For this review, take the finished solid that the model builds, in its own axes (mm). Face numbers are marked on the shaded views. A direction names the side the tool comes from. Coordinates: 2 decimals unless noted, no trailing zeros. Order: outer loops, then holes, each group sorted by start corner. A loop starts at its lowest first (then second) coordinate and runs counter-clockwise, first axis right, second up. Notation, with made-up numbers: M -6,-34.5 L 26,-34.5 A29 ccw 26,-13.5 Z; hole C 10.25,8.5 d3. An arc over 180 degrees is marked long. Use one line per item in the form item = value. Start each with the question number.
```python
from build123d import *

# Parameters (mm, degrees)
SZKIC1_W                    = 7
SZKIC1_H                    = 6
DODANIE_WYCI_GNI_CIE1_DEPTH = 0.25
SZKIC2_W                    = 7
SZKIC2_H                    = 4
DODANIE_WYCI_GNI_CIE2_DEPTH = 1.25
SZKIC3_W                    = 7
SZKIC3_H                    = 6
DODANIE_WYCI_GNI_CIE3_DEPTH = 0.5
SZKIC4_R                    = 2
DODANIE_WYCI_GNI_CIE4_DEPTH = 1.5
ZAOKR_GLENIE1_R             = 0.25
ZAOKR_GLENIE2_R             = 1
SZKIC5_W                    = 4
SZKIC5_H                    = 1
DODANIE_WYCI_GNI_CIE5_DEPTH = 1
SZKIC6_W                    = 2
SZKIC6_H                    = 0.25
WYTNIJ_WYCI_GNI_CIE1_DEPTH  = 1


with BuildPart() as part:
    # Szkic1 → Dodanie-wyciągnięcie1 (new body)
    with BuildSketch(Plane(origin=(0, 0, 0), x_dir=(1, 0, 0), z_dir=(0, 1, 0))):
        Rectangle(SZKIC1_W, SZKIC1_H)
    extrude(amount=DODANIE_WYCI_GNI_CIE1_DEPTH)

    # Szkic2 → Dodanie-wyciągnięcie2 (add)
    with BuildSketch(Plane(origin=(0, 0.25, 0), x_dir=(1, 0, 0), z_dir=(0, 1, 0))):
        Rectangle(SZKIC2_W, SZKIC2_H)
    extrude(amount=DODANIE_WYCI_GNI_CIE2_DEPTH)

    # Szkic3 → Dodanie-wyciągnięcie3 (add)
    with BuildSketch(Plane(origin=(0, 1.5, 0), x_dir=(1, 0, 0), z_dir=(0, 1, 0))):
        Rectangle(SZKIC3_W, SZKIC3_H)
    extrude(amount=DODANIE_WYCI_GNI_CIE3_DEPTH)

    # Szkic4 → Dodanie-wyciągnięcie4 (add)
    with BuildSketch(Plane(origin=(0, 2, 0), x_dir=(1, 0, 0), z_dir=(0, 1, 0))):
        with Locations(Location((0, 0, 0), (0, 0, 270))):
            Circle(SZKIC4_R)
    extrude(amount=DODANIE_WYCI_GNI_CIE4_DEPTH)

    # Zaokrąglenie1
    zaokr_glenie1_edges = [part.edges().sort_by_distance(p)[0] for p in [
        (0, 2, -2),
        (0, 3.5, -2),
    ]]
    fillet(zaokr_glenie1_edges, radius=ZAOKR_GLENIE1_R)

    # Zaokrąglenie2
    zaokr_glenie2_edges = [part.edges().sort_by_distance(p)[0] for p in [
        (-3.5, 1.75, -3),
        (3.5, 1.75, -3),
        (3.5, 1.75, 3),
        (-3.5, 1.75, 3),
    ]]
    fillet(zaokr_glenie2_edges, radius=ZAOKR_GLENIE2_R)

    # Szkic5 → Dodanie-wyciągnięcie5 (add)
    with BuildSketch(Plane.XZ):
        Rectangle(SZKIC5_W, SZKIC5_H)
    extrude(amount=DODANIE_WYCI_GNI_CIE5_DEPTH)

    # Szkic6 → Wytnij-wyciągnięcie1 (cut)
    with BuildSketch(Plane(origin=(0, 0, -0.5), x_dir=(-1, 0, 0), z_dir=(0, 0, -1))):
        with Locations((0, -0.375)):
            Rectangle(SZKIC6_W, SZKIC6_H)
    extrude(amount=-WYTNIJ_WYCI_GNI_CIE1_DEPTH, mode=Mode.SUBTRACT)


solid = part.part
```
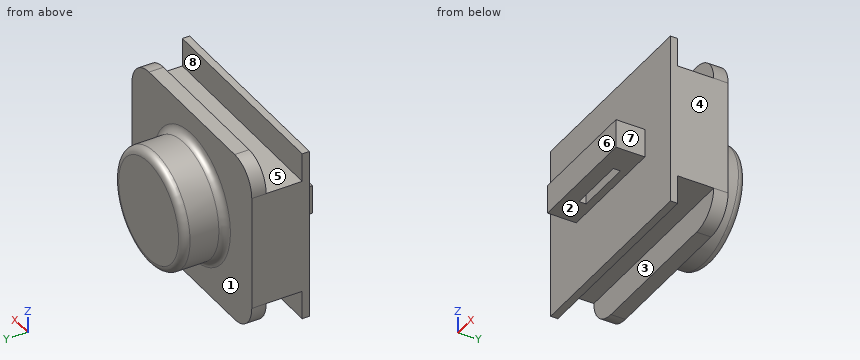
1. To check wall thickness, follow line 1 (Y direction, x = 1, z = -2.25); line 2 (Y direction, x = 0, z = -0.25); line 3 (Y direction, x = -0.25, z = 1.55). State the ranges of each line that lie inside material, in increasing order.
2. Consider section B-B, the plane y = 1.75. Write out the cut boundary in (x, z), plus the area to 3 significant figures.
3. The part is to be moulded in two halves that separate along Y. For the marked faces 6, 7 and 8, say which applies: pulls with the +Y half, pulls with the -Y half, needs draft (parallel to the pull), parting line crosses it, or undercut.
4. Consider section C-C, the plane z = 0. Write out the cut boundary in (x, y), plus the area to 3 significant figures.
5. Tool access review of the marked faces 1, 2, 3, 4 and 5: name each direction out of +Z, -Z, +X, -X, +Y, -Y from which nothing blocks a thin tool from reaching the whole face with its end or side.
6. Consider section A-A, the plane x = 0. Write out the cut boundary in (y, z).
7. For pin 1 Ø0.8 at (x, z) = (0, 2.5) entering from -Y; pin 2 Ø1 at (x, y) = (-1.5, 0.5) entering from +Z; pin 3 Ø0.8 at (x, y) = (1, -0.5) entering from -Z; pin 4 Ø0.8 at (x, z) = (1.5, 2.5) entering from +Y, all flat-tipped, find the tip position at first contact; note any pin that passes through.
8. Consider section D-D, the plane z = 2.4. Write out the cut boundary in (x, y), plus the area to 3 significant figures.
Answers follow:
q1.line_1 = 0 to 0.25, 1.5 to 2
q1.line_2 = -1 to -0.5, -0.25 to 3.5
q1.line_3 = 0 to 3.5
q2.outline = M -3.5,-2 A1 ccw -2.5,-3 L 2.5,-3 A1 ccw 3.5,-2 L 3.5,2 A1 ccw 2.5,3 L -2.5,3 A1 ccw -3.5,2 Z
q2.area = 41.1 mm²
q3.face_6 = pulls with the -Y half
q3.face_7 = needs draft
q3.face_8 = undercut
q4.outline = M -3.5,0 L -2,0 L -2,-1 L 2,-1 L 2,0 L 3.5,0 L 3.5,2 L 2.25,2 A0.25 cw 2,2.25 L 2,3.25 A0.25 ccw 1.75,3.5 L -1.75,3.5 A0.25 ccw -2,3.25 L -2,2.25 A0.25 cw -2.25,2 L -3.5,2 Z; hole M -1,-0.5 L 1,-0.5 L 1,-0.25 L -1,-0.25 Z
q4.area = 23.5 mm²
q5.face_1 = +Y
q5.face_2 = -Z, +X, -X, -Y
q5.face_3 = -Z, +X, -X
q5.face_4 = +Z, -Z, +X, +Y, -Y
q5.face_5 = +Z, +X, -X
q6.outline = M -1,-0.5 L -0.5,-0.5 L -0.5,0.5 L -1,0.5 Z; M -0.25,-0.5 L 0,-0.5 L 0,-3 L 0.25,-3 L 0.25,-2 L 1.5,-2 L 1.5,-3 L 2,-3 L 2,-2.25 A0.25 cw 2.25,-2 L 3.25,-2 A0.25 ccw 3.5,-1.75 L 3.5,1.75 A0.25 ccw 3.25,2 L 2.25,2 A0.25 cw 2,2.25 L 2,3 L 1.5,3 L 1.5,2 L 0.25,2 L 0.25,3 L 0,3 L 0,0.5 L -0.25,0.5 Z
q7.pin_1 = 0
q7.pin_2 = 3
q7.pin_3 = -0.5
q7.pin_4 = 2
q8.outline = M -3.5,0 L 3.5,0 L 3.5,0.25 L -3.5,0.25 Z; M -3.42,1.5 L 3.42,1.5 L 3.42,2 L -3.42,2 Z
q8.area = 5.17 mm²
